Read the model definition and answer for the solid it produces. Units are mm, in the model's axes. Face numbers are marked on the shaded views. Give positions to 0.01 mm unless a question says otherwise; leave off trailing zeros. Order: outer loops, then holes, each group sorted by start corner. A loop starts at its lowest first (then second) coordinate and runs counter-clockwise, first axis right, second up.
Item 1: A cutting plane is placed at A-A (z = 1.9). Write down the section's boundary in (x, y) (3 decimals), plus the area to 3 significant figures.
Item 2: A cutting plane is placed at D-D (y = 7.75). Write down the section's boundary in (x, z) (3 decimals).
Item 3: A cutting plane is placed at B-B (y = 0). Write down the section's boundary in (x, z) (3 decimals), plus the area to 3 significant figures.
Item 4: A cutting plane is placed at C-C (x = 8). Write down the section's boundary in (y, z) (3 decimals), plus the area to 3 significant figures.
Item 5: Find the intervals of material crossed by line 1 along Y through (x, z) = (-13.5, 2.5); line 2 along Y through (x, z) = (-12.5, 1.65); line 3 along X through (y, z) = (-2, 1.2), in increasing order.
Item 6: Given pin 1 Ø1.5 at (y, z) = (-5, 2.5) entering from +X, flat-ended and moving along its own axis, determine where the tip first touches the part or whether it passes through.
Item 7: The mould has two halves that part along X. Classify the marked faces 1, 2 and 3: +X half, -X half, draft (parallel to the pull), parting line (faces both ways), or undercut.
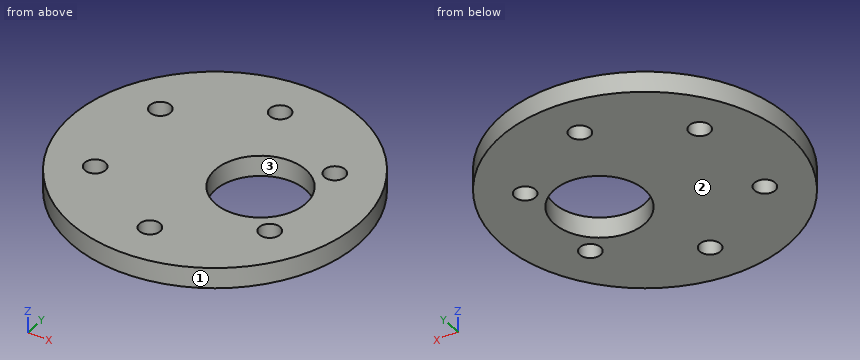
from build123d import *

# Parameters (mm, degrees)
SKETCH1_R                = 22.225
BOSS_EXTRUDE1_DEPTH      = 3.175
M3_CLEARANCE_HOLE1_D     = 3.2
M3_CLEARANCE_HOLE1_DEPTH = 3.175
CUT_EXTRUDE1_REACH       = 5.175
SKETCH4_R                = 7


with BuildPart() as part:
    # Sketch1 → Boss-Extrude1 (new body)
    with BuildSketch(Plane.XY):
        Circle(SKETCH1_R)
    extrude(amount=BOSS_EXTRUDE1_DEPTH)

    # M3 Clearance Hole1
    with Locations(Plane.XY.offset(3.175)):
        with Locations((-13.423393759, 7.75), (0, 15.5), (13.423393759, 7.75), (13.423393759, -7.75), (0, -15.5), (-13.423393759, -7.75)):
            Hole(M3_CLEARANCE_HOLE1_D / 2, depth=M3_CLEARANCE_HOLE1_DEPTH)

    # Sketch4 → Cut-Extrude1 (cut, up to next)
    with BuildSketch(Plane.XY.offset(3.175), mode=Mode.PRIVATE) as cut_extrude1_sk1:
        with Locations((7, 0)):
            Circle(SKETCH4_R)
    cut_extrude1_tool1 = extrude(cut_extrude1_sk1.sketch, amount=-CUT_EXTRUDE1_REACH, mode=Mode.PRIVATE) & part.part
    add(cut_extrude1_tool1.solids().sort_by_distance((7, 0, 3.175))[0], mode=Mode.SUBTRACT)


solid = part.part
Response values:
1. outline: circle Ø44.45 at (0, 0); hole circle Ø3.2 at (-13.423, -7.75); hole circle Ø3.2 at (-13.423, 7.75); hole circle Ø3.2 at (0, -15.5); hole circle Ø3.2 at (0, 15.5); hole circle Ø14 at (7, 0); hole circle Ø3.2 at (13.423, -7.75); hole circle Ø3.2 at (13.423, 7.75)
1. area: 1,350 mm2
2. outline: (-20.83, 0) - (-15.023, 0) - (-15.023, 3.175) - (-20.83, 3.175) - close; (-11.823, 0) - (11.823, 0) - (11.823, 3.175) - (-11.823, 3.175) - close; (15.023, 0) - (20.83, 0) - (20.83, 3.175) - (15.023, 3.175) - close
3. outline: (-22.225, 0) - (0, 0) - (0, 3.175) - (-22.225, 3.175) - close; (14, 0) - (22.225, 0) - (22.225, 3.175) - (14, 3.175) - close
3. area: 96.7 mm2
4. outline: (-20.735, 0) - (-6.928, 0) - (-6.928, 3.175) - (-20.735, 3.175) - close; (6.928, 0) - (20.735, 0) - (20.735, 3.175) - (6.928, 3.175) - close
4. area: 87.7 mm2
5. line 1: y = -17.66 to -9.35, -6.15 to 6.15, 9.35 to 17.66
5. line 2: y = -18.38 to -9.06, -6.44 to 6.44, 9.06 to 18.38
5. line 3: x = -22.13 to 0.29, 13.71 to 22.13
6. pin 1: stops at x = 21.81
7. face 1: parting line
7. face 2: draft
7. face 3: undercut
